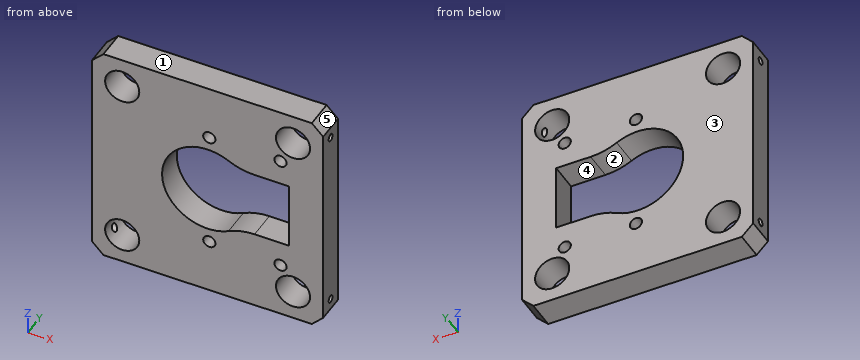
from build123d import *

# Parameters (mm, degrees)
SKETCH1_W           = 40.6
SKETCH1_H           = 40.6
BOSS_EXTRUDE1_DEPTH = 5
SKETCH2_R           = 8
CUT_EXTRUDE1_DEPTH  = 5
CUT_EXTRUDE3_DEPTH  = 6
SKETCH5_R           = 3
CUT_EXTRUDE4_DEPTH  = 10
CHAMFER1_SIZE       = 2
SKETCH6_R           = 0.65
CUT_EXTRUDE5_DEPTH  = 5
SKETCH7_R           = 0.65
CUT_EXTRUDE6_DEPTH  = 5
SKETCH8_R           = 1.075
CUT_EXTRUDE7_DEPTH  = 10
FILLET1_R           = 10


with BuildPart() as part:
    # Sketch1 → Boss-Extrude1 (new body)
    with BuildSketch(Plane(origin=(0, 0, 0), x_dir=(1, 0, 0), z_dir=(0, 1, 0))):
        Rectangle(SKETCH1_W, SKETCH1_H)
    extrude(amount=BOSS_EXTRUDE1_DEPTH)

    # Sketch2 → Cut-Extrude1 (cut)
    with BuildSketch(Plane(origin=(0, 5, 0), x_dir=(1, 0, 0), z_dir=(0, 1, 0))):
        Circle(SKETCH2_R)
    extrude(amount=-CUT_EXTRUDE1_DEPTH, mode=Mode.SUBTRACT)

    # Sketch4 → Cut-Extrude3 (cut, through all)
    with BuildSketch(Plane(origin=(0, 0, 0), x_dir=(-1, 0, 0), z_dir=(0, -1, 0))):
        Polygon((-5.291502622, 6), (-14.291502622, 6), (-14.291502622, 0), (-14.291502622, -6), (-5.291502622, -6), align=None)
    extrude(amount=-CUT_EXTRUDE3_DEPTH, mode=Mode.SUBTRACT)

    # Sketch5 → Cut-Extrude4 (cut)
    with BuildSketch(Plane(origin=(0, 5, 0), x_dir=(1, 0, 0), z_dir=(0, 1, 0))):
        with Locations((15, 15)):
            Circle(SKETCH5_R)
        with Locations((15, -15)):
            Circle(SKETCH5_R)
        with Locations((-15, -15)):
            Circle(SKETCH5_R)
        with Locations((-15, 15)):
            Circle(SKETCH5_R)
    extrude(amount=-CUT_EXTRUDE4_DEPTH, mode=Mode.SUBTRACT)

    # Chamfer1
    chamfer1_edges = [part.edges().sort_by_distance(p)[0] for p in [
        (20.3, 2.5, 20.3),
        (-20.3, 2.5, 20.3),
        (-20.3, 2.5, -20.3),
        (20.3, 2.5, -20.3),
    ]]
    chamfer(chamfer1_edges, length=CHAMFER1_SIZE)

    # Sketch6 → Cut-Extrude5 (cut)
    with BuildSketch(Plane.ZY.offset(20.3)):
        with Locations((-16.3, 2.5)):
            Circle(SKETCH6_R)
        with Locations((16.3, 2.5)):
            Circle(SKETCH6_R)
    extrude(amount=-CUT_EXTRUDE5_DEPTH, mode=Mode.SUBTRACT)

    # Sketch7 → Cut-Extrude6 (cut)
    with BuildSketch(Plane(origin=(20.3, 0, 0), x_dir=(0, 0, -1), z_dir=(1, 0, 0))):
        with Locations((16.3, 2.5)):
            Circle(SKETCH7_R)
        with Locations((-16.3, 2.5)):
            Circle(SKETCH7_R)
    extrude(amount=-CUT_EXTRUDE6_DEPTH, mode=Mode.SUBTRACT)

    # Sketch8 → Cut-Extrude7 (cut)
    with BuildSketch(Plane(origin=(0, 5, 0), x_dir=(1, 0, 0), z_dir=(0, 1, 0))):
        with Locations((0.3, -10.5)):
            Circle(SKETCH8_R)
        with Locations((12.8, -10.5)):
            Circle(SKETCH8_R)
        with Locations((0.3, 10.5)):
            Circle(SKETCH8_R)
        with Locations((12.8, 10.5)):
            Circle(SKETCH8_R)
    extrude(amount=-CUT_EXTRUDE7_DEPTH, mode=Mode.SUBTRACT)

    # Fillet1
    fillet1_edges = [part.edges().sort_by_distance(p)[0] for p in [
        (5.291502622, 2.5, -6),
        (5.291502622, 2.5, 6),
    ]]
    fillet(fillet1_edges, radius=FILLET1_R)


solid = part.part
For this review, take the finished solid that the model builds, in its own axes (mm). Face numbers are marked on the shaded views. A direction names the side the tool comes from. Round coordinates to 2 decimals unless told otherwise and drop trailing zeros. Write each loop counter-clockwise with the first axis right and the second up, starting at its lowest first coordinate (ties: lowest second). Pieces come first, ordered by that corner, then holes. Notation, with made-up numbers: (17, 19) -> (73, 19) arc R5 cw to (73, 27) -> close; hole circle Ø4 at (-16, -29.5). An arc over 180 degrees is marked (long way). Use CSV: the item, a comma, the result in double quotes.
(1) Draft analysis for pull direction Z (two halves, no side actions). For the marked faces 3, 4 and 5, state which applies: +Z half, -Z half, draft (parallel to the pull), parting line (faces both ways), or undercut.
Computed values:
face 3,"draft"
face 4,"undercut"
face 5,"+Z half"
(2) Clearance check with flat-ended pins moving along their axes: P1, Ø1.5, axis at y = 2.5, z = 16.3, coming from the +X side; P2, Ø0.8, axis at y = 2.5, z = -16.3, coming from the -X side. State where each tip first meets the part, or that it passes through.
Computed values:
P1,"x = 20.3"
P2,"x = -12.53"
(3) Consider section C-C, the plane y = 3.75. Give the number of separate pieces and of enclosed holes in the cut face, plus the area to 3 significant figures.
Computed values:
separate pieces,"1"
enclosed holes,"9"
area,"1,220 mm²"
(4) To check wall thickness, follow L1, parallel to X at y = 3.5, z = -15; L2, parallel to Z at x = 0.3, y = 2.35 (3 decimals). State the ranges of each line that lie inside material, in increasing order. Write a range as [from, to].
Computed values:
L1,"[-20.3, -18], [-12, 12], [18, 20.3]"
L2,"[-20.3, -11.575], [-9.425, -7.994], [7.994, 9.425], [11.575, 20.3]"
(5) Consider section A-A, the plane x = 15. Give the boundary of the cut face in (y, z).
Computed values:
outline,"(0, -20.3) -> (5, -20.3) -> (5, -18) -> (0, -18) -> close; (0, -12) -> (5, -12) -> (5, 12) -> (0, 12) -> close; (0, 18) -> (5, 18) -> (5, 20.3) -> (0, 20.3) -> close"
(6) Consider section D-D, the plane z = -10.5. Give the boundary of the cut face in (x, y) (3 decimals), plus the area to 4 significant figures.
Computed values:
outline,"(-20.3, 0) -> (-0.775, 0) -> (-0.775, 5) -> (-20.3, 5) -> close; (1.375, 0) -> (11.725, 0) -> (11.725, 5) -> (1.375, 5) -> close; (13.875, 0) -> (20.3, 0) -> (20.3, 5) -> (13.875, 5) -> close"
area,"181.5 mm²"
(7) Consider section B-B, the plane z = 0. Give the boundary of the cut face in (x, y), plus the area to 3 significant figures.
Computed values:
outline,"(-20.3, 0) -> (-8, 0) -> (-8, 5) -> (-20.3, 5) -> close; (14.29, 0) -> (20.3, 0) -> (20.3, 5) -> (14.29, 5) -> close"
area,"91.5 mm²"
(8) For the marked faces 1 and 2, list the 3-axis set-ups (+Z, -Z, +X, -X, +Y, -Y) from which the entire face can be reached by the end or side of a thin tool; tool diameter is ignored.
Computed values:
face 1,"+Z, +X, -X, +Y, -Y"
face 2,"+Y, -Y"
